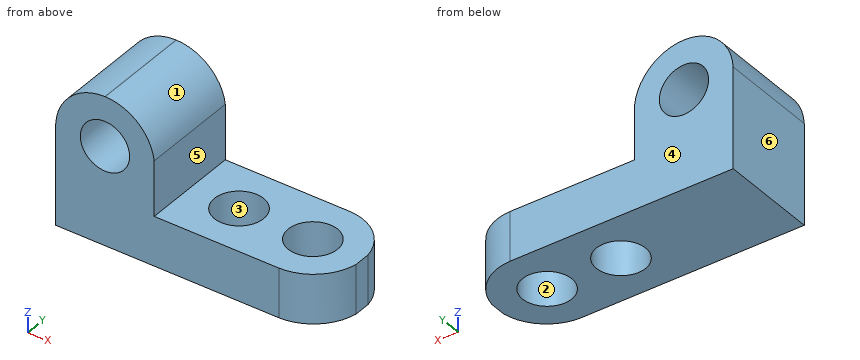
```python
from build123d import *

# Parameters (mm, degrees)
F1_DEPTH = 25.4
F2_R     = 6.35
F3_DEPTH = 25.4
F4_R     = 6.35
F5_DEPTH = 12.7


# Not quite as in the source:
# - ends of sketch curves that miss each other by under 0.0002 mm in the source are joined


with BuildPart() as f1:
    # F0 (on Front) → F1 (new body)
    with BuildSketch(Plane.XZ):
        Polygon((0, 38.1), (0, 0), (69.85, 0), (69.85, 12.7), (25.3999973736, 12.7), (25.3999973736, 38.1), align=None)
    extrude(amount=F1_DEPTH)

    # F2 (on face) → F3 (cut)
    with BuildSketch(Plane.XZ.offset(25.4)):
        with Locations((12.7, 25.4)):
            Circle(F2_R)
        with BuildLine():
            ThreePointArc((12.7392116615, 38.1000602784), (21.1944094362, 34.8947951162), (25.3999973736, 26.8899763006))
            Line((25.3999973736, 26.8899763006), (25.3999973736, 38.1))
            Line((25.3999973736, 38.1), (12.7392116615, 38.1000602784))
        make_face()
        with BuildLine():
            ThreePointArc((0, 25.9728431702), (3.9449392563, 34.5834780061), (12.7392116615, 38.1000602784))
            Line((12.7392116615, 38.1000602784), (0, 38.1))
            Line((0, 38.1), (0, 25.9728431702))
        make_face()
    extrude(amount=-F3_DEPTH, mode=Mode.SUBTRACT)

    # F4 (on face) → F5 (cut)
    with BuildSketch(Plane.XY.offset(12.7)):
        with Locations((38.1, -12.7)):
            Circle(F4_R)
        with Locations((57.15, -12.7)):
            Circle(F4_R)
        with BuildLine():
            ThreePointArc((57.5116686145, 0), (65.5882036204, -3.0491682704), (69.85, -10.5568267911))
            Line((69.85, -10.5568267911), (69.85, 0))
            Line((69.85, 0), (57.5116686145, 0))
        make_face()
        with BuildLine():
            ThreePointArc((69.85, -14.8431732089), (65.5882036204, -22.3508317296), (57.5116686145, -25.4))
            Line((57.5116686145, -25.4), (69.85, -25.4))
            Line((69.85, -25.4), (69.85, -14.8431732089))
        make_face()
    extrude(amount=-F5_DEPTH, mode=Mode.SUBTRACT)


solid = f1.part
```
The model under review builds one solid part; all positions refer to its coordinate system, in mm. Face numbers are marked on the shaded views. A direction names the side the tool comes from. Round coordinates to 2 decimals unless told otherwise and drop trailing zeros. Loops run counter-clockwise (first coordinate to the right, second up) from the corner with the lowest first, then second, coordinate; pieces in that order, holes last. Notation, with made-up numbers: (64, 44.5) -> (117, 44.5) arc R25 cw to (117, 65.5) -> close; hole circle Ø5 at (54, -7.75). An arc over 180 degrees is marked (long way). Answer in a Markdown table with one row per item.
1) For pin 1 Ø8 at (y, z) = (-3, 4.5) entering from +X; pin 2 Ø11.5 at (x, z) = (12.7, 25.4) entering from +Y; pin 3 Ø12.5 at (x, y) = (54.5, -8) entering from +Z; pin 4 Ø6 at (y, z) = (-4, 17.5) entering from +X, all flat-tipped, find the tip position at first contact; note any pin that passes through.
Taken from the geometry:
| item | result |
|---|---|
| pin 1 | stops at x = 68.68 |
| pin 2 | passes through |
| pin 3 | stops at z = 12.7 |
| pin 4 | stops at x = 25.4 |
2) Consider section B-B, the plane x = 38.1. Write out the cut boundary in (y, z), plus the area to 3 significant figures.
Taken from the geometry:
| item | result |
|---|---|
| outline | (-25.4, 0) -> (-19.05, 0) -> (-19.05, 12.7) -> (-25.4, 12.7) -> close; (-6.35, 0) -> (0, 0) -> (0, 12.7) -> (-6.35, 12.7) -> close |
| area | 161 mm² |
3) Tool access review of the marked faces 5 and 6: name each direction out of +Z, -Z, +X, -X, +Y, -Y from which nothing blocks a thin tool from reaching the whole face with its end or side.
Taken from the geometry:
| item | result |
|---|---|
| face 5 | +Z, +X, +Y, -Y |
| face 6 | +Z, -Z, -X, +Y, -Y |
4) Wall thickness on line 1 along X through (y, z) = (-18.5, 10.5); line 2 along Z through (x, y) = (12.7, -13.5); line 3 along Y through (x, z) = (38.1, 4): over which ranges is each line inside the solid? List them lowest first.
Taken from the geometry:
| item | result |
|---|---|
| line 1 | x = 0 to 35.51, 40.69 to 54.56, 59.74 to 68.63 |
| line 2 | z = 0 to 19.05, 31.75 to 38.1 |
| line 3 | y = -25.4 to -19.05, -6.35 to 0 |
5) Consider section A-A, the plane y = -12.7. Write out the cut boundary in (x, z).
Taken from the geometry:
| item | result |
|---|---|
| outline | (0, 0) -> (31.75, 0) -> (31.75, 12.7) -> (25.4, 12.7) -> (25.4, 26.89) arc R12.75 ccw to (12.78, 38.1) -> (12.7, 38.1) arc R12.75 ccw to (0, 25.97) -> close; (44.45, 0) -> (50.8, 0) -> (50.8, 12.7) -> (44.45, 12.7) -> close; (63.5, 0) -> (69.85, 0) -> (69.85, 12.7) -> (63.5, 12.7) -> close; hole circle Ø12.7 at (12.7, 25.4) |
6) Consider section C-C, the plane z = 10. Write out the cut boundary in (x, y), plus the area to 3 significant figures.
Taken from the geometry:
| item | result |
|---|---|
| outline | (0, -25.4) -> (57.51, -25.4) arc R12.7 ccw to (69.85, -14.84) -> (69.85, -10.56) arc R12.7 ccw to (57.51, 0) -> (0, 0) -> close; hole circle Ø12.7 at (38.1, -12.7); hole circle Ø12.7 at (57.15, -12.7) |
| area | 1,460 mm² |
7) Consider section D-D, the plane z = 22. Write out the cut boundary in (x, y), plus the area to 3 significant figures.
Taken from the geometry:
| item | result |
|---|---|
| outline | (0, -25.4) -> (7.34, -25.4) -> (7.34, 0) -> (0, 0) -> close; (18.06, -25.4) -> (25.4, -25.4) -> (25.4, 0) -> (18.06, 0) -> close |
| area | 373 mm² |
8) Draft analysis for pull direction Y (two halves, no side actions). For the marked faces 1, 2, 3 and 4, state which applies: pulls with the +Y half, pulls with the -Y half, needs draft (parallel to the pull), parting line crosses it, or undercut.
Taken from the geometry:
| item | result |
|---|---|
| face 1 | needs draft |
| face 2 | undercut |
| face 3 | undercut |
| face 4 | pulls with the +Y half |
